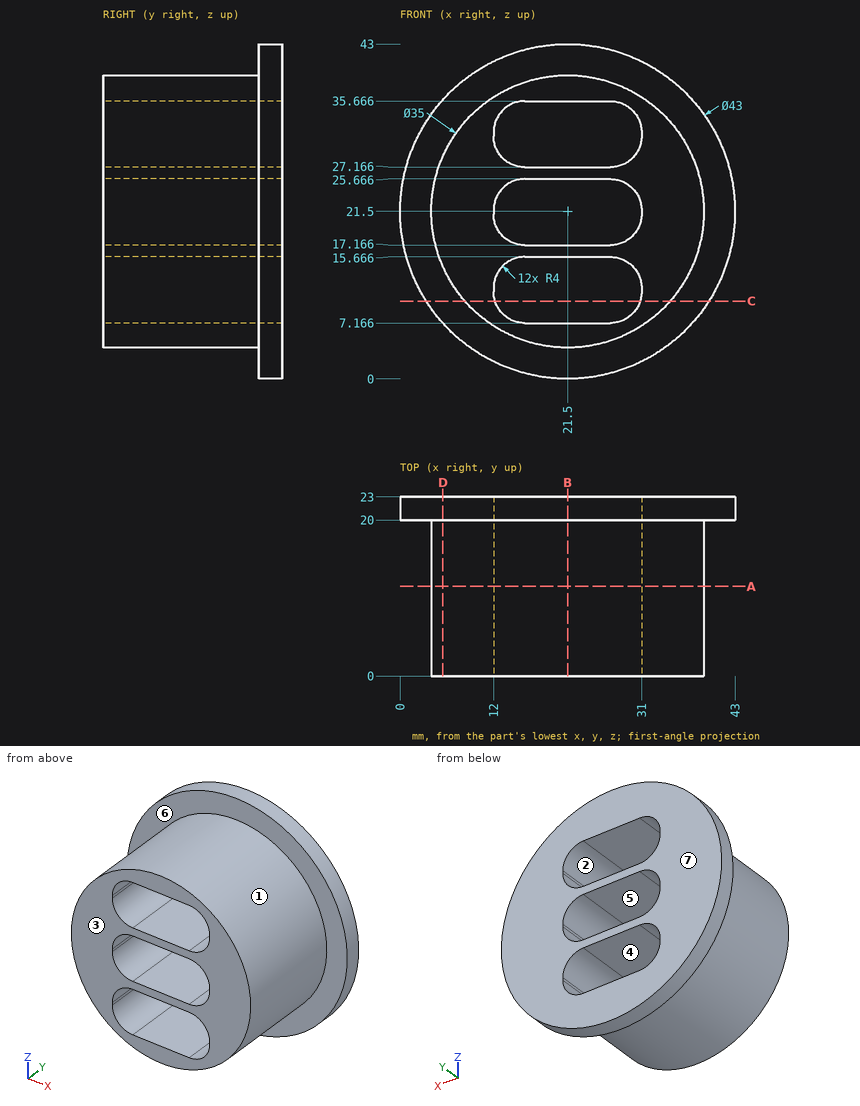
Drawing for the job (mm, zero at the part's lowest x, y, z). A direction names the side the tool comes from. Give positions to 0.01 mm unless a question says otherwise; leave off trailing zeros. Loops run counter-clockwise (first coordinate to the right, second up) from the corner with the lowest first, then second, coordinate; pieces in that order, holes last.
(1) Band-saw the part on A-A (y = 11.5). Write the cut outline in (x, z).
Return value:
outline: circle Ø35 at (21.5, 21.5); hole (12, 11.17) arc R4 ccw to (16, 7.17) - (27, 7.17) arc R4 ccw to (31, 11.17) - (31, 11.67) arc R4 ccw to (27, 15.67) - (16, 15.67) arc R4 ccw to (12, 11.67) - close; hole (12, 21.17) arc R4 ccw to (16, 17.17) - (27, 17.17) arc R4 ccw to (31, 21.17) - (31, 21.67) arc R4 ccw to (27, 25.67) - (16, 25.67) arc R4 ccw to (12, 21.67) - close; hole (12, 31.17) arc R4 ccw to (16, 27.17) - (27, 27.17) arc R4 ccw to (31, 31.17) - (31, 31.67) arc R4 ccw to (27, 35.67) - (16, 35.67) arc R4 ccw to (12, 31.67) - close
(2) Drill centre lines: line 1 along Z through (x, y) = (15, 12); line 2 along Z through (x, y) = (29, 5); line 3 along X through (y, z) = (13, 34). Where is each one in solid material? Low to high.
Return value:
line 1: z = 5.25 to 7.29, 15.54 to 17.29, 25.54 to 27.29, 35.54 to 37.75
line 2: z = 5.69 to 7.7, 15.13 to 17.7, 25.13 to 27.7, 35.13 to 37.31
line 3: x = 9.25 to 12.75, 30.25 to 33.75
(3) Band-saw the part on D-D (x = 5.5). Write the cut outline in (y, z), and give its area (3 significant figures).
Return value:
outline: (0, 14.41) - (20, 14.41) - (20, 7.14) - (23, 7.14) - (23, 35.86) - (20, 35.86) - (20, 28.59) - (0, 28.59) - close
area: 370 mm2
(4) Pull direction X, two halves, no side cores. Call the marked faces 1, 2, 3 and 4: pulls with the +X half, pulls with the -X half, needs draft (parallel to the pull), parting line crosses it, or undercut.
Return value:
face 1: parting line crosses it
face 2: undercut
face 3: needs draft
face 4: undercut
(5) 3-axis set-ups, long thin cutter, end or side, ignore diameter. For the marked faces 5, 6 and 7: which of +Z, -Z, +X, -X, +Y, -Y reach the whole face in a straight line?
Return value:
face 5: +Y, -Y
face 6: -Y
face 7: +Z, -Z, +X, -X, +Y
(6) Band-saw the part on C-C (z = 10). Write the cut outline in (x, y), and give its area (3 significant figures).
Return value:
outline: (3.33, 20) - (8.31, 20) - (8.31, 0) - (12.17, 0) - (12.17, 23) - (3.33, 23) - close; (30.83, 0) - (34.69, 0) - (34.69, 20) - (39.67, 20) - (39.67, 23) - (30.83, 23) - close
area: 208 mm2
(7) Band-saw the part on B-B (x = 21.5). Write the cut outline in (y, z).
Return value:
outline: (0, 4) - (20, 4) - (20, 0) - (23, 0) - (23, 7.17) - (0, 7.17) - close; (0, 15.67) - (23, 15.67) - (23, 17.17) - (0, 17.17) - close; (0, 25.67) - (23, 25.67) - (23, 27.17) - (0, 27.17) - close; (0, 35.67) - (23, 35.67) - (23, 43) - (20, 43) - (20, 39) - (0, 39) - close
(8) Pin check, flat tips, straight feed: pin 1 (9 mm diameter, centred on x = 23.5, y = 13.5, fed in from +Z); pin 2 (12 mm diameter, centred on x = 22, y = 9, fed in from -Z); pin 3 (8 mm diameter, centred on x = 21, y = 18, fed in from +Z); pin 4 (10 mm diameter, centred on y = 6.5, z = 25.5, fed in from +X). Stop position of each tip, or through.
Return value:
pin 1: stops at z = 39
pin 2: stops at z = 4
pin 3: stops at z = 43
pin 4: stops at x = 39
